from build123d import *

# Parameters (mm, degrees)
SKETCH3_R          = 5
CUT_EXTRUDE1_DEPTH = 63.261545114
CIRPATTERN1_COUNT  = 4


with BuildPart() as part:
    # Sketch2 → Revolve1 (revolve)
    with BuildSketch(Plane.XY, mode=Mode.PRIVATE) as revolve1_sk:
        Polygon((11.25, 0), (11.25, 12), (19, 12), (26.323794171, 42), (32.5, 42), (22.246688161, 0), align=None)
    revolve(revolve1_sk.sketch.rotate(Axis((0, 0, 0), (0, 1, 0)), 90), axis=Axis((0, 0, 0), (0, 1, 0)))

    # Sketch3 → Cut-Extrude1 (cut, symmetric)
    with BuildSketch(Plane.XY):
        with Locations((0, 42)):
            Circle(SKETCH3_R)
    cut_extrude1 = extrude(amount=CUT_EXTRUDE1_DEPTH, both=True, mode=Mode.SUBTRACT)

    # CirPattern1: Cut-Extrude1 ×4 about axis
    cirpattern1_axis = Axis((0, 0, 0), (0, -1, 0))
    for i in range(1, CIRPATTERN1_COUNT):
        add(cut_extrude1.rotate(cirpattern1_axis, i * 360 / CIRPATTERN1_COUNT), mode=Mode.SUBTRACT)


solid = part.part
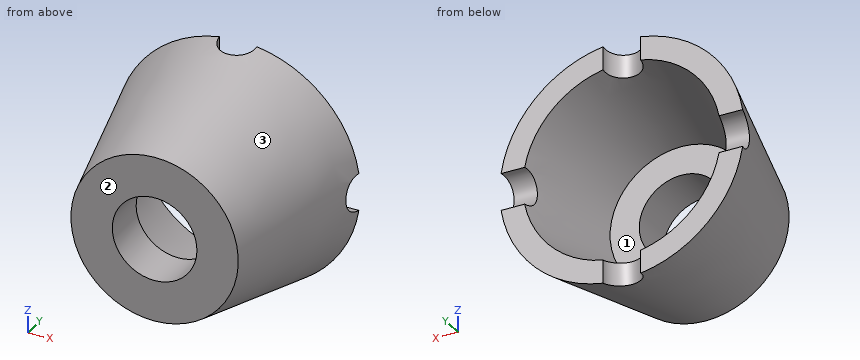
CAD build for the part. Positions are in the model's coordinates, mm. Face numbers are marked on the shaded views. Give positions to 0.01 mm unless a question says otherwise; leave off trailing zeros. Order: outer loops, then holes, each group sorted by start corner. A loop starts at its lowest first (then second) coordinate and runs counter-clockwise, first axis right, second up. Notation, with made-up numbers: (63, 38.5) -> (85, 38.5) arc R15 cw to (85, 45.5) -> close; hole circle Ø4 at (-13, -9.5). An arc over 180 degrees is marked (long way). Return JSON: item names as keys, results as strings.
Q1. Drill centre lines: line 1 (X direction, y = 30, z = -4); line 2 (X direction, y = 20.5, z = 17.5); line 3 (Z direction, x = 18.5, y = 21). Where is each one in solid material? Low to high.
Working result:
{"line 1": "-29.3 to -23.05, 23.05 to 29.3", "line 2": "-20.89 to -11.74, 11.74 to 20.89", "line 3": "-20.18 to -10.35, 10.35 to 20.18"}
Q2. Saw through at A-A (z = 0). Write the cut outline in (x, y), then the cut area to 3 significant figures.
Working result:
{"outline": "(-31.28, 37) -> (-22.25, 0) -> (-11.25, 0) -> (-11.25, 12) -> (-19, 12) -> (-25.1, 37) -> close; (11.25, 0) -> (22.25, 0) -> (31.28, 37) -> (25.1, 37) -> (19, 12) -> (11.25, 12) -> close", "area": "608 mm²"}
Q3. Mould opens along Z. For the marked faces 1, 2 and 3 say: pulls with the +Z half, pulls with the -Z half, needs draft (parallel to the pull), parting line crosses it, or undercut.
Working result:
{"face 1": "undercut", "face 2": "needs draft", "face 3": "parting line crosses it"}
Q4. Saw through at B-B (x = 0). Write the cut outline in (y, z), then the cut area to 3 significant figures.
Working result:
{"outline": "(0, -22.25) -> (37, -31.28) -> (37, -25.1) -> (12, -19) -> (12, -11.25) -> (0, -11.25) -> close; (0, 11.25) -> (12, 11.25) -> (12, 19) -> (37, 25.1) -> (37, 31.28) -> (0, 22.25) -> close", "area": "608 mm²"}
Q5. Flat gauge pins, fed straight in: pin 1 (12 mm diameter, centred on y = 10, z = -3.5, fed in from -X); pin 2 (8 mm diameter, centred on x = 23, z = 5.5, fed in from +Y); pin 3 (1 mm diameter, centred on y = 22, z = 11, fed in from -X); pin 4 (1.5 mm diameter, centred on y = 6.5, z = 2.5, fed in from +X). Where does each tip first touch, or does it go through?
Working result:
{"pin 1": "x = -26.03", "pin 2": "y = 42", "pin 3": "x = -25.58", "pin 4": "x = 23.9"}
Q6. Saw through at C-C (y = 20). Write the cut outline in (x, z), then the cut area to 3 significant figures.
Working result:
{"outline": "circle Ø54.26 at (0, 0); hole circle Ø41.91 at (0, 0)", "area": "933 mm²"}
